The model under review builds one solid part; all positions refer to its coordinate system, in mm. Face numbers are marked on the shaded views. A direction names the side the tool comes from. Coordinates: 2 decimals unless noted, no trailing zeros. Loops run counter-clockwise (first coordinate to the right, second up) from the corner with the lowest first, then second, coordinate; pieces in that order, holes last. Notation, with made-up numbers: (21, -15) - (47, -15) arc R13 cw to (47, 10) - close; hole circle Ø8 at (-30, -2.75). An arc over 180 degrees is marked (long way). Use a Markdown table: item, result. Add a question column.
1) For the marked faces 1, 2, 3 and 4, list the 3-axis set-ups (+Z, -Z, +X, -X, +Y, -Y) from which the entire face can be reached by the end or side of a thin tool; tool diameter is ignored.
2) Add section B-B, the plane x = -24. Give the boundary of the cut face in (y, z), and give its area (3 significant figures).
3) Add section A-A, the plane z = 0. Give the boundary of the cut face in (x, y), and give its area (3 significant figures).
4) Add section D-D, the plane x = 26.5. Give the boundary of the cut face in (y, z), and give its area (3 significant figures).
5) To check wall thickness, follow L1, parallel to Z at x = 1, y = 14.5; L2, parallel to Z at x = 21.5, y = 13.5; L3, parallel to Y at x = 23, z = 13.5. State the ranges of each line that lie inside material, in increasing order. Write a range as [from, to].
6) Add section C-C, the plane y = 3.25. Give the boundary of the cut face in (x, z), and give its area (3 significant figures).
7) Clearance check with flat-ended pins moving along their axes: pin 1 (3 mm diameter, centred on y = 14.5, z = 30, fed in from -X); pin 2 (0.5 mm diameter, centred on x = -5, y = 15.5, fed in from -Z); pin 3 (1.5 mm diameter, centred on x = -9.5, y = 14, fed in from -Z). State where each tip first meets the part, or that it passes through.
8) The part is to be moulded in two halves that separate along Z. For the marked faces 5 and 6, say which applies: pulls with the +Z half, pulls with the -Z half, needs draft (parallel to the pull), parting line crosses it, or undercut.
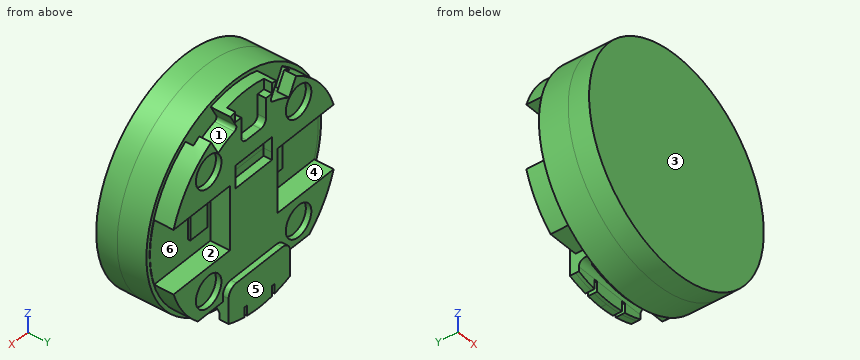
```python
from build123d import *

# Parameters (mm, degrees)
SKETCH1_R           = 33.52
BOSS_EXTRUDE1_DEPTH = 9
SKETCH2_R           = 32.29
BOSS_EXTRUDE2_DEPTH = 6.12
CUT_EXTRUDE1_START  = -6
CUT_EXTRUDE1_DEPTH  = 6
SKETCH10_R          = 2
CUT_EXTRUDE2_DEPTH  = 59.369629946
SKETCH23_W          = 6.054526745
SKETCH23_H          = 4
CUT_EXTRUDE3_DEPTH  = 59.369629972
BOSS_EXTRUDE4_DEPTH = 1.78
CUT_EXTRUDE5_START  = -6
CUT_EXTRUDE5_DEPTH  = 6
CUT_EXTRUDE6_START  = -2.54
SKETCH26_W          = 14
SKETCH26_H          = 4.621469047
CUT_EXTRUDE6_DEPTH  = 2.54
CUT_EXTRUDE7_START  = -6.12
CUT_EXTRUDE7_DEPTH  = 6.12
SKETCH26_7_R        = 4.9
CUT_EXTRUDE8_DEPTH  = 1.7
SKETCH37_W          = 5.66557495
SKETCH37_H          = 2.46
CUT_EXTRUDE13_DEPTH = 2.7
SKETCH30_W          = 5.66557495
SKETCH30_H          = 2.46
CUT_EXTRUDE14_DEPTH = 2.7
SKETCH40_W          = 6.5
SKETCH40_H          = 8
BOSS_EXTRUDE5_DEPTH = 0.68
CUT_EXTRUDE15_START = -4.1
CUT_EXTRUDE15_DEPTH = 4.1
BOSS_EXTRUDE6_START = 6.44
SKETCH41_R          = 33.52
BOSS_EXTRUDE6_DEPTH = 6.44
SKETCH43_W          = 14
SKETCH43_H          = 2.54
CUT_EXTRUDE16_DEPTH = 2.44
FILLET1_R           = 1
FILLET2_R           = 1


with BuildPart() as part:
    # Sketch1 → Boss-Extrude1 (new body)
    with BuildSketch(Plane(origin=(0, 0, 0), x_dir=(1, 0, 0), z_dir=(0, 1, 0))):
        with Locations(Location((0, 0, 0), (0, 0, 270))):
            Circle(SKETCH1_R)
    extrude(amount=BOSS_EXTRUDE1_DEPTH)

    # Sketch2 → Boss-Extrude2 (add)
    with BuildSketch(Plane(origin=(0, 9, 0), x_dir=(1, 0, 0), z_dir=(0, 1, 0))):
        with Locations(Location((0, 0, 0), (0, 0, 270))):
            Circle(SKETCH2_R)
    extrude(amount=BOSS_EXTRUDE2_DEPTH)

    # Sketch3 → Cut-Extrude1 (cut)
    with BuildSketch(Plane(origin=(0, 15.12, 0), x_dir=(1, 0, 0), z_dir=(0, 1, 0)).offset(CUT_EXTRUDE1_START)):
        with BuildLine():
            Line((-11.81, 24.153658108), (-11.81, 30.052753618))
            ThreePointArc((-11.81, 30.052753618), (-16.879698811, 27.5267119), (-21.43, 24.153658108))
            Line((-21.43, 24.153658108), (-11.81, 24.153658108))
        make_face()
        with BuildLine():
            ThreePointArc((21.43, 24.153658108), (16.879698811, 27.5267119), (11.81, 30.052753618))
            Line((11.81, 30.052753618), (11.81, 24.153658108))
            Line((11.81, 24.153658108), (21.43, 24.153658108))
        make_face()
    extrude(amount=CUT_EXTRUDE1_DEPTH, mode=Mode.SUBTRACT)

    # Sketch10 → Cut-Extrude2 (cut, through all)
    with BuildSketch(Plane.ZY.offset(11.81)):
        with Locations(Location((-28.653658108, 12.12, 0), (0, 0, 134.390731556))):
            Circle(SKETCH10_R)
    extrude(amount=-CUT_EXTRUDE2_DEPTH, mode=Mode.SUBTRACT)

    # Sketch23 → Cut-Extrude3 (cut, through all)
    with BuildSketch(Plane.ZY.offset(11.81)):
        with Locations((-31.680921481, 12.12)):
            Rectangle(SKETCH23_W, SKETCH23_H)
    extrude(amount=-CUT_EXTRUDE3_DEPTH, mode=Mode.SUBTRACT)

    # Sketch24 → Boss-Extrude4 (add)
    with BuildSketch(Plane(origin=(0, 15.12, 0), x_dir=(1, 0, 0), z_dir=(0, 1, 0))):
        with BuildLine():
            ThreePointArc((0, 32.29), (-6.010020203, 31.725758575), (-11.81, 30.052753618))
            Line((-11.81, 30.052753618), (-11.81, 24.153658108))
            Line((-11.81, 24.153658108), (-11.81, 22.29))
            ThreePointArc((-11.81, 22.29), (-10.931320344, 20.168679656), (-8.81, 19.29))
            Line((-8.81, 19.29), (0, 19.29))
            Line((0, 19.29), (0, 32.29))
        make_face()
        with BuildLine():
            ThreePointArc((11.81, 30.052753618), (6.010020203, 31.725758575), (0, 32.29))
            Line((0, 32.29), (0, 19.29))
            Line((0, 19.29), (8.81, 19.29))
            ThreePointArc((8.81, 19.29), (10.931320344, 20.168679656), (11.81, 22.29))
            Line((11.81, 22.29), (11.81, 24.153658108))
            Line((11.81, 24.153658108), (11.81, 30.052753618))
        make_face()
    extrude(amount=BOSS_EXTRUDE4_DEPTH)

    # Sketch26<4> → Cut-Extrude5 (cut)
    with BuildSketch(Plane(origin=(0, 15.12, 0), x_dir=(1, 0, 0), z_dir=(0, 1, 0)).offset(CUT_EXTRUDE5_START)):
        with BuildLine():
            ThreePointArc((30.718749975, -9.95), (32.29, 0), (30.718749975, 9.95))
            Line((30.718749975, 9.95), (9.138749975, 9.95))
            Line((9.138749975, 9.95), (9.138749975, -9.95))
            Line((9.138749975, -9.95), (30.718749975, -9.95))
        make_face()
    cut_extrude5 = extrude(amount=CUT_EXTRUDE5_DEPTH, mode=Mode.SUBTRACT)

    # Sketch26 → Cut-Extrude6 (cut)
    with BuildSketch(Plane(origin=(0, 15.12, 0), x_dir=(1, 0, 0), z_dir=(0, 1, 0)).offset(CUT_EXTRUDE6_START)):
        with BuildLine():
            ThreePointArc((-7.1, -31.499747618), (0, -32.29), (7.1, -31.499747618))
            Line((7.1, -31.499747618), (7.1, -28.259676136))
            Line((7.1, -28.259676136), (4.74, -28.259676136))
            Line((4.74, -28.259676136), (4.74, -26.204757202))
            Line((4.74, -26.204757202), (4.74, -22.05))
            ThreePointArc((4.74, -22.05), (4.154213562, -20.635786438), (2.74, -20.05))
            Line((2.74, -20.05), (-2.74, -20.05))
            ThreePointArc((-2.74, -20.05), (-4.154213562, -20.635786438), (-4.74, -22.05))
            Line((-4.74, -22.05), (-4.74, -26.204757202))
            Line((-4.74, -26.204757202), (-4.74, -28.259676136))
            Line((-4.74, -28.259676136), (-7.1, -28.259676136))
            Line((-7.1, -28.259676136), (-7.1, -31.499747618))
        make_face()
        with Locations((0, -12.539265477)):
            Rectangle(SKETCH26_W, SKETCH26_H)
    extrude(amount=CUT_EXTRUDE6_DEPTH, mode=Mode.SUBTRACT)

    # Sketch28 → Cut-Extrude7 (cut)
    with BuildSketch(Plane(origin=(0, 15.12, 0), x_dir=(1, 0, 0), z_dir=(0, 1, 0)).offset(CUT_EXTRUDE7_START)):
        with BuildLine():
            ThreePointArc((-6.138643472, -25.91281452), (-9.99763899, -24.682060583), (-13.62533551, -22.880278238))
            Line((-13.62533551, -22.880278238), (-16.282957683, -27.883855348))
            ThreePointArc((-16.282957683, -27.883855348), (-12.673955944, -29.698736349), (-8.866590913, -31.048794913))
            Line((-8.866590913, -31.048794913), (-6.138643472, -25.91281452))
        make_face()
        with BuildLine():
            ThreePointArc((13.62533551, -22.880278238), (9.99763899, -24.682060583), (6.138643472, -25.91281452))
            Line((6.138643472, -25.91281452), (8.866590913, -31.048794913))
            ThreePointArc((8.866590913, -31.048794913), (12.673955944, -29.698736349), (16.282957683, -27.883855348))
            Line((16.282957683, -27.883855348), (13.62533551, -22.880278238))
        make_face()
    extrude(amount=CUT_EXTRUDE7_DEPTH, mode=Mode.SUBTRACT)

    # Sketch26<7> → Cut-Extrude8 (cut)
    with BuildSketch(Plane(origin=(0, 15.12, 0), x_dir=(1, 0, 0), z_dir=(0, 1, 0))):
        with Locations(Location((17.253376134, 17.489232673, 0), (0, 0, 270))):
            Circle(SKETCH26_7_R)
        with Locations(Location((17.253376134, -19.410767327, 0), (0, 0, 270))):
            Circle(SKETCH26_7_R)
        with Locations(Location((-17.253376134, -19.410767327, 0), (0, 0, 270))):
            Circle(SKETCH26_7_R)
        with Locations(Location((-17.253376134, 17.489232673, 0), (0, 0, 270))):
            Circle(SKETCH26_7_R)
    extrude(amount=-CUT_EXTRUDE8_DEPTH, mode=Mode.SUBTRACT)

    # Sketch37 → Cut-Extrude13 (cut)
    with BuildSketch(Plane(origin=(1.148573691, 0, -0.610058532), x_dir=(0.4690825196866177, 0, 0.8831543408286312), z_dir=(-0.8831543408286312, 0, 0.4690825196866177))):
        with Locations((29.431011233, 10.23)):
            Rectangle(SKETCH37_W, SKETCH37_H)
    extrude(amount=-CUT_EXTRUDE13_DEPTH, mode=Mode.SUBTRACT)

    # Sketch30 → Cut-Extrude14 (cut)
    with BuildSketch(Plane(origin=(-1.148573691, 0, -0.610058532), x_dir=(0.4690825196866177, 0, -0.8831543408286312), z_dir=(0.8831543408286312, 0, 0.4690825196866177))):
        with Locations((-29.431011233, 10.23)):
            Rectangle(SKETCH30_W, SKETCH30_H)
    extrude(amount=-CUT_EXTRUDE14_DEPTH, mode=Mode.SUBTRACT)

    # Sketch40 → Boss-Extrude5 (add)
    with BuildSketch(Plane(origin=(0, 9.12, 0), x_dir=(1, 0, 0), z_dir=(0, 1, 0))):
        with Locations((14.388749975, 0.25)):
            Rectangle(SKETCH40_W, SKETCH40_H)
    boss_extrude5 = extrude(amount=BOSS_EXTRUDE5_DEPTH)

    # Sketch31 → Cut-Extrude15 (cut)
    with BuildSketch(Plane(origin=(0, 16.9, 0), x_dir=(1, 0, 0), z_dir=(0, 1, 0)).offset(CUT_EXTRUDE15_START)):
        with BuildLine():
            ThreePointArc((-4.81, 31.929735358), (-5.310654422, 31.850291201), (-5.81, 31.76299734))
            Line((-5.81, 31.76299734), (-5.81, 28.77))
            Line((-5.81, 28.77), (-4.81, 28.77))
            Line((-4.81, 28.77), (-4.81, 31.929735358))
        make_face()
        with BuildLine():
            ThreePointArc((5.81, 31.76299734), (5.310654422, 31.850291201), (4.81, 31.929735358))
            Line((4.81, 31.929735358), (4.81, 28.77))
            Line((4.81, 28.77), (5.81, 28.77))
            Line((5.81, 28.77), (5.81, 31.76299734))
        make_face()
    extrude(amount=CUT_EXTRUDE15_DEPTH, mode=Mode.SUBTRACT)

    # Sketch41 → Boss-Extrude6 (add)
    with BuildSketch(Plane.XZ.offset(BOSS_EXTRUDE6_START)):
        with Locations(Location((0, 0, 0), (0, 0, 270))):
            Circle(SKETCH41_R)
    extrude(amount=-BOSS_EXTRUDE6_DEPTH)

    # Sketch43 → Cut-Extrude16 (cut)
    with BuildSketch(Plane.XY.offset(10.228530953)):
        with Locations((0, 13.85)):
            Rectangle(SKETCH43_W, SKETCH43_H)
    extrude(amount=-CUT_EXTRUDE16_DEPTH, mode=Mode.SUBTRACT)

    # Mirror1: Cut-Extrude5 across plane
    add(cut_extrude5.mirror(Plane.ZY), mode=Mode.SUBTRACT)

    # Mirror2: Boss-Extrude5 across plane
    add(boss_extrude5.mirror(Plane.ZY))

    # Fillet1
    fillet1_edges = [part.edges().sort_by_distance(p)[0] for p in [
        (6.138643472, 12.06, 25.91281452),
    ]]
    fillet(fillet1_edges, radius=FILLET1_R)

    # Fillet2
    fillet2_edges = [part.edges().sort_by_distance(p)[0] for p in [
        (-6.138643472, 12.06, 25.91281452),
    ]]
    fillet(fillet2_edges, radius=FILLET2_R)


solid = part.part
```
From the geometry:
| question | item | result |
|---|---|---|
| 1 | face 1 | +Y |
| 1 | face 2 | +X, +Y |
| 1 | face 3 | +Z, -Z, +X, -X, -Y |
| 1 | face 4 | -X, +Y |
| 2 | outline | (-6.44, -23.4) - (9, -23.4) - (9, -21.6) - (15.12, -21.6) - (15.12, -9.95) - (9.12, -9.95) - (9.12, 9.95) - (15.12, 9.95) - (15.12, 21.6) - (9, 21.6) - (9, 23.4) - (-6.44, 23.4) - close |
| 2 | area | 868 mm^2 |
| 3 | outline | (-33.52, -6.44) - (33.52, -6.44) - (33.52, 9) - (32.29, 9) - (32.29, 9.12) - (17.64, 9.12) - (17.64, 9.8) - (11.14, 9.8) - (11.14, 9.12) - (9.14, 9.12) - (9.14, 15.12) - (-9.14, 15.12) - (-9.14, 9.12) - (-11.14, 9.12) - (-11.14, 9.8) - (-17.64, 9.8) - (-17.64, 9.12) - (-32.29, 9.12) - (-32.29, 9) - (-33.52, 9) - close |
| 3 | area | 1,160 mm^2 |
| 4 | outline | (-6.44, -20.53) - (9, -20.53) - (9, -18.45) - (15.12, -18.45) - (15.12, -9.95) - (9.12, -9.95) - (9.12, 9.95) - (15.12, 9.95) - (15.12, 18.45) - (9, 18.45) - (9, 20.53) - (-6.44, 20.53) - close |
| 4 | area | 740 mm^2 |
| 5 | L1 | z = [-32.27, 7.79], [14.85, 20.05] |
| 5 | L2 | z = [-24.09, -19.93], [-15.04, -9.95], [9.95, 16.97], [21.86, 24.09] |
| 5 | L3 | y = [-6.44, 15.12] |
| 6 | outline | circle Ø67.04 at (0, 0) |
| 6 | area | 3,530 mm^2 |
| 7 | pin 1 | stops at x = -8.87 |
| 7 | pin 2 | stops at z = -31.94 |
| 7 | pin 3 | stops at z = -31.08 |
| 8 | face 5 | needs draft |
| 8 | face 6 | undercut |
